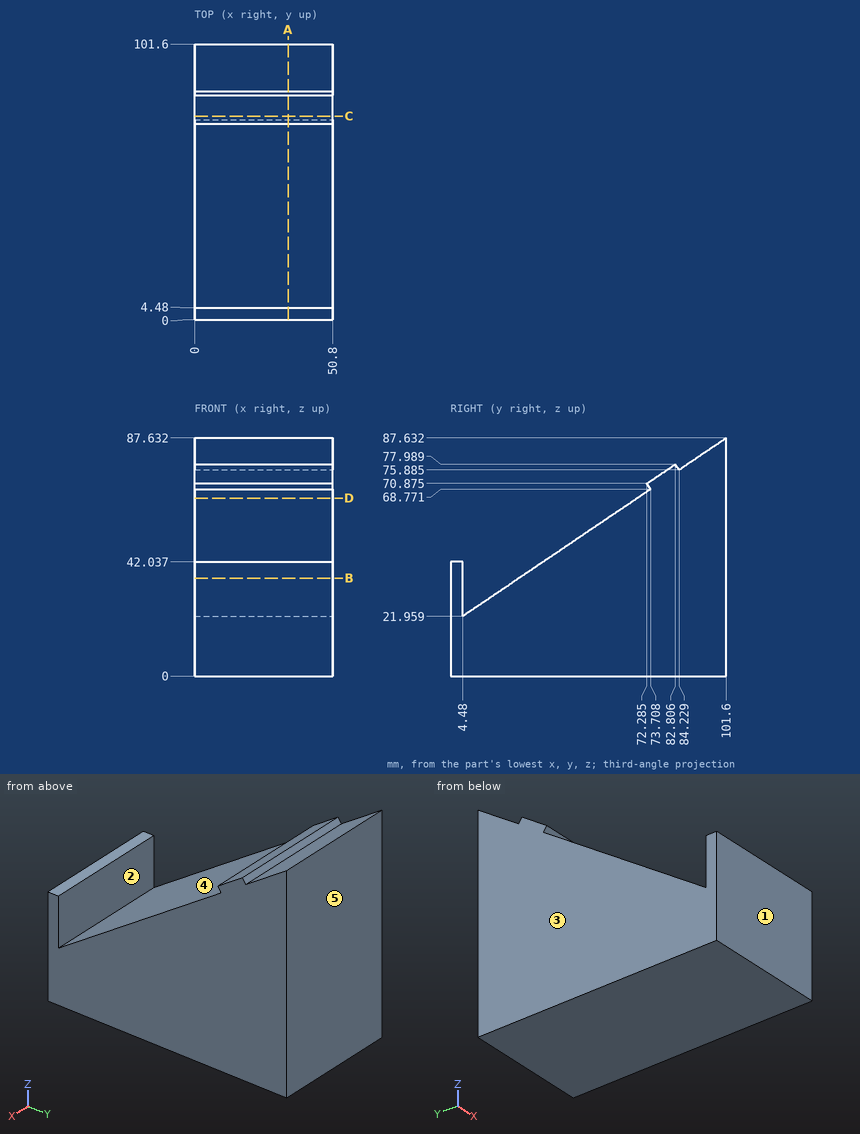
Input: dimensioned drawing with shaded views. Units: mm. Origin: part minimum x, y, z. A direction names the side the tool comes from. Round coordinates to 2 decimals unless told otherwise and drop trailing zeros. Order: outer loops, then holes, each group sorted by start corner. A loop starts at its lowest first (then second) coordinate and runs counter-clockwise, first axis right, second up. Notation, with made-up numbers: M 76,-16 L 89,-16 A20 ccw 89,3 Z; hole C -17.5,30 d8. An arc over 180 degrees is marked long. Use one line per item in the form item = value. Start each with the question number.
Q1. Pin query (flat end, axial travel): pin 1 Ø1 at (x, y) = (22.5, 48) entering from +Z (1 decimal); pin 2 Ø1 at (x, z) = (22.5, 48) entering from -Y; pin 3 Ø1.3 at (x, y) = (15, 3) entering from +Z. Return the tip coordinate at first contact, or that it passes through.
Q2. Cut plane A-A (x = 34.5). Return loops of the section in (y, z) (1 decimal).
Q3. Cut plane B-B (z = 36). Return loops of the section in (x, y) (1 decimal).
Q4. Mould query, pull axis Y, two halves, no side actions, for the marked faces 3, 4 and 5. Classes: +Y half, -Y half, draft (parallel to the pull), parting line (faces both ways), or undercut.
Q5. Cut plane D-D (z = 65.5). Return loops of the section in (x, y), and give its area (3 significant figures).
Q6. Material intervals for line 1 (Y direction, x = 34.5, z = 32); line 2 (Y direction, x = 18, z = 40); line 3 (Z direction, x = 28, y = 35) (1 decimal), sorted ascending. Write a range as [from, to].
Q7. Cut plane C-C (y = 75). Return loops of the section in (x, z), and give its area (3 significant figures).
Q8. Access query for the marked faces 1 and 2. Directions: +Z, -Z, +X, -X, +Y, -Y. A direction counts if a zero-diameter tool reaches every point of the face in a straight line with its end or side. Return the directions, or none.
Geometry results:
q1.pin_1 = 51.7
q1.pin_2 = 42.25
q1.pin_3 = 42.04
q2.outline = M 0,0 L 101.6,0 L 101.6,87.6 L 84.2,75.9 L 82.8,78 L 72.3,70.9 L 73.7,68.8 L 4.5,22 L 4.5,42 L 0,42 Z
q3.outline = M 0,0 L 50.8,0 L 50.8,4.5 L 0,4.5 Z; M 0,25.2 L 50.8,25.2 L 50.8,101.6 L 0,101.6 Z
q4.face_3 = draft
q4.face_4 = undercut
q4.face_5 = +Y half
q5.outline = M 0,68.87 L 50.8,68.87 L 50.8,101.6 L 0,101.6 Z
q5.area = 1,660 mm^2
q6.line_1 = [0, 4.48], [19.33, 101.6]
q6.line_2 = [0, 4.48], [31.16, 101.6]
q6.line_3 = [0, 42.6]
q7.outline = M 0,0 L 50.8,0 L 50.8,72.71 L 0,72.71 Z
q7.area = 3,690 mm^2
q8.face_1 = +Z, -Z, +X, -X, -Y
q8.face_2 = +Z, +X, -X
